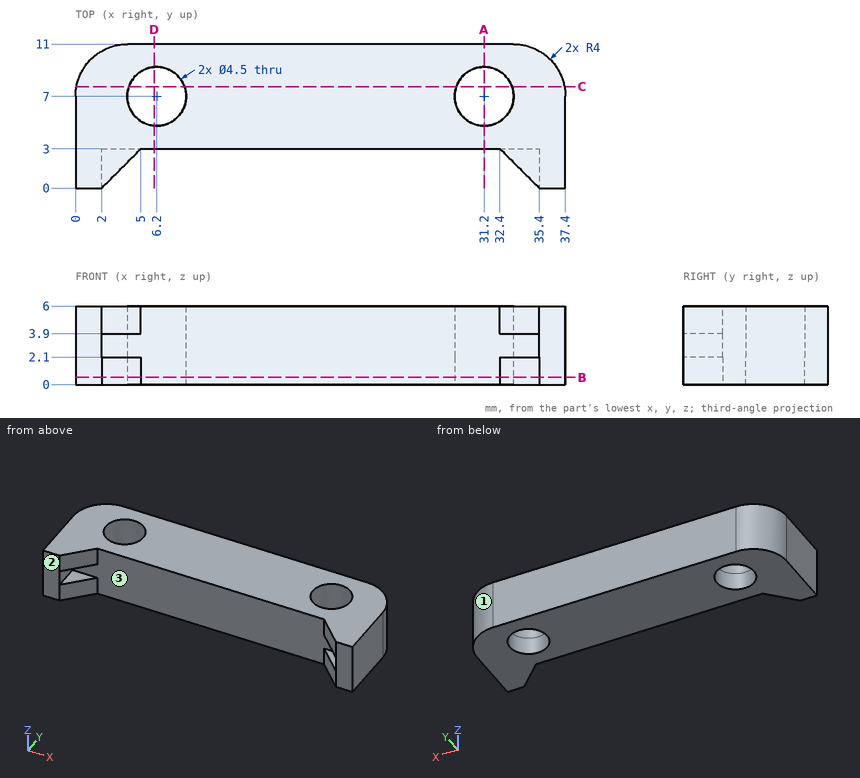
Study the drawing (mm; zero at the part's minimum x, y, z) and answer. Coordinates: 2 decimals unless noted, no trailing zeros. Write each loop counter-clockwise with the first axis right and the second up, starting at its lowest first coordinate (ties: lowest second). Pieces come first, ordered by that corner, then holes.
Q1. A cutting plane is placed at A-A, the plane x = 31.2. Give the vertices of the cut face in (y, z).
Q2. Each of these flat-tipped pins is pushed along its axis until it touches: pin 1 Ø2.5 at (x, y) = (6.2, 7) entering from -Z; pin 2 Ø3 at (x, z) = (13.5, 0.5) entering from -Y. Where does it stop, or does it pass through?
Q3. A cutting plane is placed at B-B, the plane z = 0.55. Give the vertices of the cut face in (x, y), then the cut area to 3 significant figures.
Q4. Determine the mould class of the marked faces 1, 2 and 3 for opening direction X: released by +X, released by -X, zero draft, split by the parting line, or undercut.
Q5. A cutting plane is placed at C-C, the plane y = 7.75. Give the vertices of the cut face in (x, z).
Q6. Find the intervals of material crossed by line 1 (X direction, y = 7, z = 1); line 2 (X direction, y = 2, z = 4.1); line 3 (Y direction, x = 6.2, z = 0.85), in increasing order.
Q7. A cutting plane is placed at D-D, the plane x = 6. Give the vertices of the cut face in (y, z), then the cut area to 3 significant figures.
Findings below:
1. outline: (3, 0) - (4.75, 0) - (4.75, 6) - (3, 6) - close; (9.25, 0) - (11, 0) - (11, 6) - (9.25, 6) - close
2. pin 1: passes through
2. pin 2: stops at y = 3
3. outline: (0, 0) - (2, 0) - (5, 3) - (32.4, 3) - (35.4, 0) - (37.4, 0) - (37.4, 7) arc R4 ccw to (33.4, 11) - (4, 11) arc R4 ccw to (0, 7) - close; hole circle Ø4.5 at (6.2, 7); hole circle Ø4.5 at (31.2, 7)
3. area: 282 mm2
4. face 1: released by +X
4. face 2: zero draft
4. face 3: undercut
5. outline: (0.07, 0) - (4.08, 0) - (4.08, 6) - (0.07, 6) - close; (8.32, 0) - (29.08, 0) - (29.08, 6) - (8.32, 6) - close; (33.32, 0) - (37.33, 0) - (37.33, 6) - (33.32, 6) - close
6. line 1: x = 0 to 3.95, 8.45 to 28.95, 33.45 to 37.4
6. line 2: x = 0 to 4, 33.4 to 37.4
6. line 3: y = 3 to 4.75, 9.25 to 11
7. outline: (3, 0) - (4.76, 0) - (4.76, 6) - (3, 6) - close; (9.24, 0) - (11, 0) - (11, 6) - (9.24, 6) - close
7. area: 21.1 mm2
